Can you work these out from the model? Positions are in its coordinate system, mm. A direction names the side the tool comes from. Round coordinates to 2 decimals unless told otherwise and drop trailing zeros. Loops run counter-clockwise (first coordinate to the right, second up) from the corner with the lowest first, then second, coordinate; pieces in that order, holes last.
from build123d import *

# Parameters (mm, degrees)
SKETCH1_R           = 60.75
SKETCH1_R_2         = 59.75
BOSS_EXTRUDE1_DEPTH = 21
SKETCH2_R           = 60.75
BOSS_EXTRUDE2_DEPTH = 2
SKETCH3_R           = 1.6
BOSS_EXTRUDE3_DEPTH = 2


with BuildPart() as part:
    # Sketch1 → Boss-Extrude1 (new body)
    with BuildSketch(Plane(origin=(0, 0, 0), x_dir=(1, 0, 0), z_dir=(0, 1, 0))):
        with Locations(Location((0, 0, 0), (0, 0, 90))):
            Circle(SKETCH1_R)
        with Locations(Location((0, 0, 0), (0, 0, 90))):
            Circle(SKETCH1_R_2, mode=Mode.SUBTRACT)
    extrude(amount=BOSS_EXTRUDE1_DEPTH)

    # Sketch2 → Boss-Extrude2 (add)
    with BuildSketch(Plane(origin=(0, 21, 0), x_dir=(1, 0, 0), z_dir=(0, 1, 0))):
        with Locations(Location((0, 0, 0), (0, 0, 90))):
            Circle(SKETCH2_R)
    extrude(amount=BOSS_EXTRUDE2_DEPTH)

    # Sketch3 → Boss-Extrude3 (add)
    # profile 1 of 4: a face of its own
    with BuildSketch(Plane(origin=(0, 0, 0), x_dir=(1, 0, 0), z_dir=(0, 1, 0))):
        with BuildLine():
            Line((5, 66.893889039), (5, 60.543889039))
            Line((5, 60.543889039), (-5, 60.543889039))
            Line((-5, 60.543889039), (-5, 66.893889039))
            ThreePointArc((-5, 66.893889039), (0, 71.893889039), (5, 66.893889039))
        make_face()
        with Locations(Location((0, 66.893889039, 0), (0, 0, 270))):
            Circle(SKETCH3_R, mode=Mode.SUBTRACT)
    # profile 2 of 4: a face of its own
    with BuildSketch(Plane(origin=(0, 0, 0), x_dir=(1, 0, 0), z_dir=(0, 1, 0))):
        with BuildLine():
            Line((60.543889039, 5), (66.893889039, 5))
            ThreePointArc((66.893889039, 5), (71.893889039, 0), (66.893889039, -5))
            Line((66.893889039, -5), (60.543889039, -5))
            Line((60.543889039, -5), (60.543889039, 5))
        make_face()
        with Locations(Location((66.893889039, 0, 0), (0, 0, 270))):
            Circle(SKETCH3_R, mode=Mode.SUBTRACT)
    # profile 3 of 4: a face of its own
    with BuildSketch(Plane(origin=(0, 0, 0), x_dir=(1, 0, 0), z_dir=(0, 1, 0))):
        with BuildLine():
            Line((5, -60.543889039), (5, -66.893889039))
            ThreePointArc((5, -66.893889039), (0, -71.893889039), (-5, -66.893889039))
            Line((-5, -66.893889039), (-5, -60.543889039))
            Line((-5, -60.543889039), (5, -60.543889039))
        make_face()
        with Locations(Location((0, -66.893889039, 0), (0, 0, 270))):
            Circle(SKETCH3_R, mode=Mode.SUBTRACT)
    # profile 4 of 4: a face of its own
    with BuildSketch(Plane(origin=(0, 0, 0), x_dir=(1, 0, 0), z_dir=(0, 1, 0))):
        with BuildLine():
            Line((-60.543889039, -5), (-66.893889039, -5))
            ThreePointArc((-66.893889039, -5), (-71.893889039, 0), (-66.893889039, 5))
            Line((-66.893889039, 5), (-60.543889039, 5))
            Line((-60.543889039, 5), (-60.543889039, -5))
        make_face()
        with Locations(Location((-66.893889039, 0, 0), (0, 0, 270))):
            Circle(SKETCH3_R, mode=Mode.SUBTRACT)
    extrude(amount=BOSS_EXTRUDE3_DEPTH)


solid = part.part
(1) If I drill on line 1 (X direction, y = 1.4, z = 0); line 2 (X direction, y = 19.75, z = 0.5); line 3 (Y direction, x = 30, z = 31.5), over which ranges is the centre line in solid material (lowest first)?
Worked answers:
line 1: x = -71.89 to -68.49, -65.29 to -59.75, 59.75 to 65.29, 68.49 to 71.89
line 2: x = -60.75 to -59.75, 59.75 to 60.75
line 3: y = 21 to 23
(2) For faces 1 (the cylindrical face through (22.885, 10.353, -55.194)), 2 (the cylindrical face through (0.07, 0.986, -68.492)), which set-ups out of +Z, -Z, +X, -X, +Y, -Y let a thin tool reach every point of the face, with its end or its side?
Worked answers:
face 1: -Y
face 2: +Y, -Y
(3) Will these pins go through, and if not, where does the flat tip stop? P1, Ø8, axis at x = 1, z = 68, coming from the +Y side; P2, Ø2, axis at x = -49, y = 6, coming from the +Z side; P3, Ø2, axis at x = 63.5, y = 1, coming from the -Z side; P4, Ø2.5, axis at x = 0, z = -66.89, coming from the +Y side.
Worked answers:
P1: stops at y = 2
P2: stops at z = 37.24
P3: stops at z = -5
P4: passes through
(4) If we section it at B-B, the plane x = 43.5: List the corners of the cut face in (y, z) for me.
Worked answers:
outline: (0, -42.41) - (23, -42.41) - (23, 42.41) - (0, 42.41) - (0, 40.96) - (21, 40.96) - (21, -40.96) - (0, -40.96) - close
(5) If we section it at A-A, the plane y = 11: List the corners of the cut face in (x, z) for me.
Worked answers:
outline: circle Ø121.5 at (0, 0); hole circle Ø119.5 at (0, 0)
(6) If we section it at C-C, the plane z = -49: List the corners of the cut face in (x, y) for me.
Worked answers:
outline: (-35.91, 0) - (-34.19, 0) - (-34.19, 21) - (34.19, 21) - (34.19, 0) - (35.91, 0) - (35.91, 23) - (-35.91, 23) - close
(7) If we mould it in two halves opening along Z, with no side actions, what happens to faces 3 (the cylindrical face through (-0.613, 0.986, 68.372)), 4 (the flat face through (-1, 23, 1)), 5 (the cylindrical face through (0.11, 0.986, 71.893)), 6 (the cylindrical face through (23.268, 11.339, -56.118))? For each: released by +Z, released by -Z, zero draft, split by the parting line, or undercut.
Worked answers:
face 3: undercut
face 4: zero draft
face 5: released by +Z
face 6: split by the parting line
